Can you work these out from the model? Positions are in its coordinate system, mm. Coordinates: 2 decimals unless noted, no trailing zeros. Order: outer loops, then holes, each group sorted by start corner. A loop starts at its lowest first (then second) coordinate and runs counter-clockwise, first axis right, second up. Notation, with made-up numbers: M 2,89 L 57,89 A15 cw 57,98 Z; hole C 60,-14.75 d4. An arc over 180 degrees is marked long. Answer as CSV lines item,"result". Start each with the question number.
1. Will these pins go through, and if not, where does the flat tip stop? pin 1 (1 mm diameter, centred on y = 272, z = 1, fed in from -X); pin 2 (1 mm diameter, centred on y = 288, z = 0.5, fed in from +X).
2. If we section it at B-B (x = 150): List the corners of the cut face in (y, z) for me.
3. If we section it at C-C (y = 112): List the corners of the cut face in (x, z) for me, plus the area to 3 significant figures.
4. If we section it at A-A (z = 0.4): Give the number of separate pieces and of enclosed holes in the cut face, plus the area to 3 significant figures.
5. If we section it at D-D (x = 116): List the corners of the cut face in (y, z) for me.
6. I need wall thicknesses on line 1 along Y through (x, z) = (150, 1.4); line 2 along Y through (x, z) = (67, 1.05); line 3 along X through (y, z) = (38.5, 0.65). Which ranges of each line are inside material? Lowest first, please. Write a range as from..to.
```python
from build123d import *

# Parameters (mm, degrees)
AUFSATZ_LINEAR_AUSTRAGEN1_DEPTH                      = 2
FORMSENKUNG_F_R_M4_SENKSCHRAUBE_MIT_INNE_D           = 4.5
FORMSENKUNG_F_R_M4_SENKSCHRAUBE_MIT_INNE_DEPTH       = 15
FORMSENKUNG_F_R_M4_SENKSCHRAUBE_MIT_INNE_CSINK_D     = 8.6
FORMSENKUNG_F_R_M4_SENKSCHRAUBE_MIT_INNE_CSINK_ANGLE = 90
FORMSENKUNG_F_R_M4_SENKSCHRAUBE_MIT_INNE_TIP         = 1.351936393
SKIZZE4_R                                            = 95
SCHNITT_LINEAR_AUSTRAGEN1_DEPTH                      = 10
ERDUNG_AT_2_COUNT                                    = 2
ERDUNG_AT_2_PITCH                                    = 204.963132201
SKIZZE7_W                                            = 234
SKIZZE7_H                                            = 8
SCHNITT_LINEAR_AUSTRAGEN2_DEPTH                      = 10
VERRUNDUNG1_R                                        = 4


with BuildPart() as part:
    # Skizze1 → Aufsatz-Linear austragen1 (new body)
    with BuildSketch(Plane.XY):
        Polygon((0, 0), (300, 0), (300, 23), (277, 23), (277, 440), (300, 440), (300, 470), (0, 470), (0, 440), (23, 440), (23, 23), (0, 23), align=None)
    extrude(amount=AUFSATZ_LINEAR_AUSTRAGEN1_DEPTH)

    # Formsenkung für M4 Senkschraube mit Innensechskant1
    with Locations(Plane.XY.offset(2)):
        with Locations((292, 11.5), (8, 11.5), (11.5, 455), (288.5, 455)):
            CounterSinkHole(FORMSENKUNG_F_R_M4_SENKSCHRAUBE_MIT_INNE_D / 2, FORMSENKUNG_F_R_M4_SENKSCHRAUBE_MIT_INNE_CSINK_D / 2, depth=FORMSENKUNG_F_R_M4_SENKSCHRAUBE_MIT_INNE_DEPTH, counter_sink_angle=FORMSENKUNG_F_R_M4_SENKSCHRAUBE_MIT_INNE_CSINK_ANGLE)
            with Locations((0, 0, -(FORMSENKUNG_F_R_M4_SENKSCHRAUBE_MIT_INNE_DEPTH + FORMSENKUNG_F_R_M4_SENKSCHRAUBE_MIT_INNE_TIP / 2))):  # 118° drill point
                Cone(0, FORMSENKUNG_F_R_M4_SENKSCHRAUBE_MIT_INNE_D / 2, FORMSENKUNG_F_R_M4_SENKSCHRAUBE_MIT_INNE_TIP, mode=Mode.SUBTRACT)

    # Skizze4 → Schnitt-Linear austragen1 (cut)
    with BuildSketch(Plane.XY.offset(2)):
        with Locations((150, 112)):
            Circle(SKIZZE4_R)
    extrude(amount=-SCHNITT_LINEAR_AUSTRAGEN1_DEPTH, mode=Mode.SUBTRACT)

    # Skizze6 → Erdung (revolve, cut)
    with BuildSketch(Plane(origin=(60, 450, 2), x_dir=(0, -1, 0), z_dir=(1, 0, 0))):
        Polygon((0, 0), (0, 2), (2.25, 2), (2.25, 2.05), (4.3, 0), align=None)
    erdung = revolve(axis=Axis((60, 450, 8.35), (0, 0, -1)), mode=Mode.SUBTRACT)

    # Erdung at 2: Erdung ×2
    with Locations(*[Vector(-0.17833221510322264, 0.9839703354554842, 0) * (i * ERDUNG_AT_2_PITCH) for i in range(1, ERDUNG_AT_2_COUNT)]):
        add(erdung, mode=Mode.SUBTRACT)

    # Skizze7 → Schnitt-Linear austragen2 (cut)
    with BuildSketch(Plane(origin=(0, 0, 0), x_dir=(-1, 0, 0), z_dir=(0, 0, -1))):
        with Locations((-150, 246)):
            Rectangle(SKIZZE7_W, SKIZZE7_H)
    extrude(amount=-SCHNITT_LINEAR_AUSTRAGEN2_DEPTH, mode=Mode.SUBTRACT)

    # Verrundung1
    verrundung1_edges = [part.edges().sort_by_distance(p)[0] for p in [
        (33, 242, 1),
        (33, 250, 1),
        (267, 242, 1),
        (267, 250, 1),
    ]]
    fillet(verrundung1_edges, radius=VERRUNDUNG1_R - 0.0001)  # a hair under: the kernel refuses the full size


solid = part.part
```
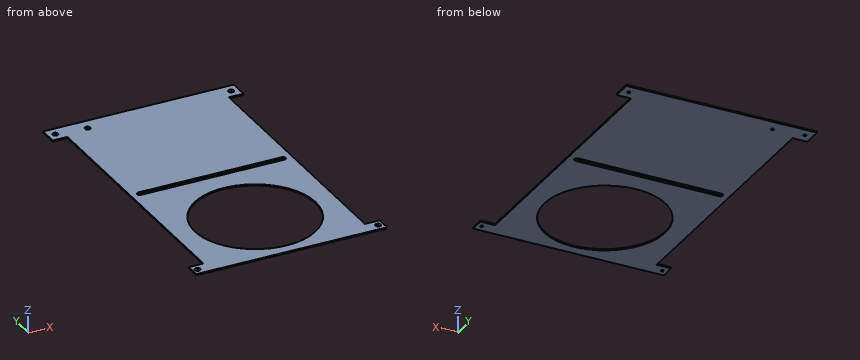
Solved:
1,pin 1,"x = 23"
1,pin 2,"x = 277"
2,outline,"M 0,0 L 17,0 L 17,2 L 0,2 Z; M 207,0 L 242,0 L 242,2 L 207,2 Z; M 250,0 L 470,0 L 470,2 L 250,2 Z"
3,outline,"M 23,0 L 55,0 L 55,2 L 23,2 Z; M 245,0 L 277,0 L 277,2 L 245,2 Z"
3,area,"128 mm²"
4,separate pieces,"1"
4,enclosed holes,"7"
4,area,"91,500 mm²"
5,outline,"M 0,0 L 23.29,0 L 23.29,2 L 0,2 Z; M 200.71,0 L 242,0 L 242,2 L 200.71,2 Z; M 250,0 L 470,0 L 470,2 L 250,2 Z"
6,line 1,"0..17, 207..242, 250..470"
6,line 2,"0..65.78, 158.22..242, 250..470"
6,line 3,"23..89.81, 210.19..277"
